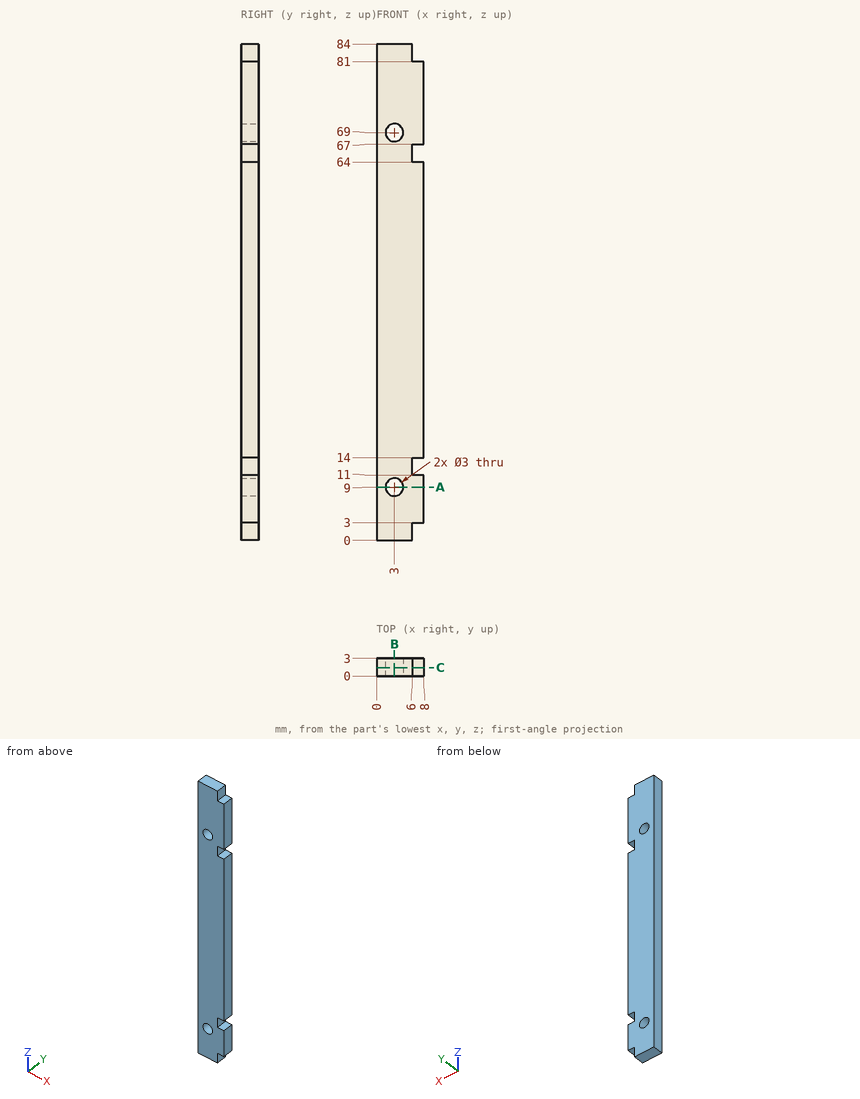
Answer from the drawing. Dimensions are ordinates in mm from the lowest x, y and z of the part. Coordinates: 2 decimals unless noted, no trailing zeros. Write each loop counter-clockwise with the first axis right and the second up, starting at its lowest first coordinate (ties: lowest second). Pieces come first, ordered by that corner, then holes. Notation, with made-up numbers: M 58.25,2 L 102.25,2 A24 ccw 102.25,38 Z; hole C -26,-7 d4. An arc over 180 degrees is marked long. Write item = value, one per line.
1. Straight lines are drawn through the part: line 1 (Z direction, x = 3, y = 1.85); line 2 (Z direction, x = 6.75, y = 0.5); line 3 (X direction, y = 1.25, z = 69). For each, find the intervals that lie inside material, in ascending order. Write a range as from..to.
Solution:
line_1 = 0..7.5, 10.5..67.5, 70.5..84
line_2 = 3..11, 14..64, 67..81
line_3 = 0..1.5, 4.5..8
2. Flat-ended cylindrical pins translate along their axes: pin 1 (0.6 mm diameter, centred on x = 7, y = 2, fed in from +Z); pin 2 (1 mm diameter, centred on x = 7, y = 1, fed in from -Z); pin 3 (0.9 mm diameter, centred on y = 1, z = 12, fed in from +X); pin 4 (1.5 mm diameter, centred on y = 2.5, z = 69, fed in from -X). Find the tip coordinate at first contact, or state that the pin passes through.
Solution:
pin_1 = 81
pin_2 = 3
pin_3 = 6
pin_4 = 0
3. The part is cut by section A-A (z = 9). Determine the outline of the cut face in (x, y).
Solution:
outline = M 0,0 L 1.5,0 L 1.5,3 L 0,3 Z; M 4.5,0 L 8,0 L 8,3 L 4.5,3 Z
4. The part is cut by section C-C (y = 1.4). Determine the outline of the cut face in (x, z).
Solution:
outline = M 0,0 L 6,0 L 6,3 L 8,3 L 8,11 L 6,11 L 6,14 L 8,14 L 8,64 L 6,64 L 6,67 L 8,67 L 8,81 L 6,81 L 6,84 L 0,84 Z; hole C 3,9 d3; hole C 3,69 d3
5. The part is cut by section B-B (x = 3). Determine the outline of the cut face in (y, z), then the cut area to 3 significant figures.
Solution:
outline = M 0,0 L 3,0 L 3,7.5 L 0,7.5 Z; M 0,10.5 L 3,10.5 L 3,67.5 L 0,67.5 Z; M 0,70.5 L 3,70.5 L 3,84 L 0,84 Z
area = 234 mm2
